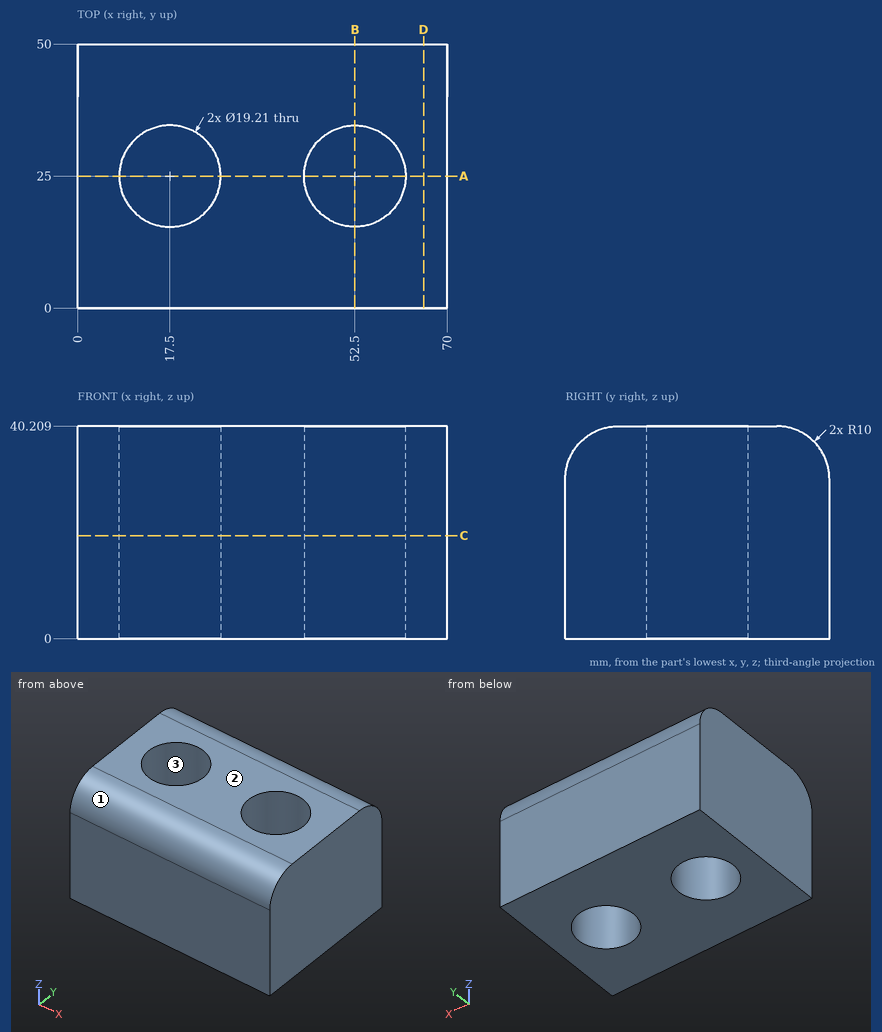
Input: dimensioned drawing with shaded views. Units: mm. Origin: part minimum x, y, z. Give positions to 0.01 mm unless a question says otherwise; leave off trailing zeros. Write each loop counter-clockwise with the first axis right and the second up, starting at its lowest first coordinate (ties: lowest second). Pieces come first, ordered by that corner, then holes. Notation, with made-up numbers: (-17, 28) -> (18, 28) arc R21 cw to (18, 56) -> close; hole circle Ø7 at (42, 49). An arc over 180 degrees is marked (long way). Return JSON: item names as keys, results as strings. Group by question number.
1. Section B-B, the plane x = 52.5. Output: boundary loops of the cut face in (y, z) (1 decimal).
2. Section D-D, the plane x = 65.5. Output: boundary loops of the cut face in (y, z).
3. Mould query, pull axis Y, two halves, no side actions, for the marked faces 1, 2 and 3. Classes: +Y half, -Y half, draft (parallel to the pull), parting line (faces both ways), or undercut.
4. Section C-C, the plane z = 19.5. Output: boundary loops of the cut face in (x, y) (1 decimal), then the cut area to 3 significant figures.
5. Material intervals for line 1 (Y direction, x = 52.5, z = 13) (1 decimal); line 2 (X direction, y = 18, z = 17.5) (1 decimal); line 3 (X direction, y = 31, z = 11), sorted ascending. Write a range as from..to.
6. Section A-A, the plane y = 25. Output: boundary loops of the cut face in (x, z) (1 decimal).
7. Pin query (flat end, axial travel): pin 1 Ø1.5 at (y, z) = (44.5, 4) entering from -X; pin 2 Ø1 at (x, y) = (38.5, 42.5) entering from +Z. Return the tip coordinate at first contact, or that it passes through.
Determined:
{
 "1": {"outline": "(0, 0) -> (15.4, 0) -> (15.4, 40.2) -> (10, 40.2) arc R10 ccw to (0, 30.2) -> close; (34.6, 0) -> (50, 0) -> (50, 30.2) arc R10 ccw to (40, 40.2) -> (34.6, 40.2) -> close"},
 "2": {"outline": "(0, 0) -> (50, 0) -> (50, 30.21) arc R10 ccw to (40, 40.21) -> (10, 40.21) arc R10 ccw to (0, 30.21) -> close"},
 "3": {"face 1": "-Y half", "face 2": "draft", "face 3": "undercut"},
 "4": {"outline": "(0, 0) -> (70, 0) -> (70, 50) -> (0, 50) -> close; hole circle Ø19.2 at (17.5, 25); hole circle Ø19.2 at (52.5, 25)", "area": "2,920 mm2"},
 "5": {"line 1": "y = 0..15.4, 34.6..50", "line 2": "x = 0..10.9, 24.1..45.9, 59.1..70", "line 3": "x = 0..10, 25..45, 60..70"},
 "6": {"outline": "(0, 0) -> (7.9, 0) -> (7.9, 40.2) -> (0, 40.2) -> close; (27.1, 0) -> (42.9, 0) -> (42.9, 40.2) -> (27.1, 40.2) -> close; (62.1, 0) -> (70, 0) -> (70, 40.2) -> (62.1, 40.2) -> close"},
 "7": {"pin 1": "stops at x = 0", "pin 2": "stops at z = 40.01"}
}
